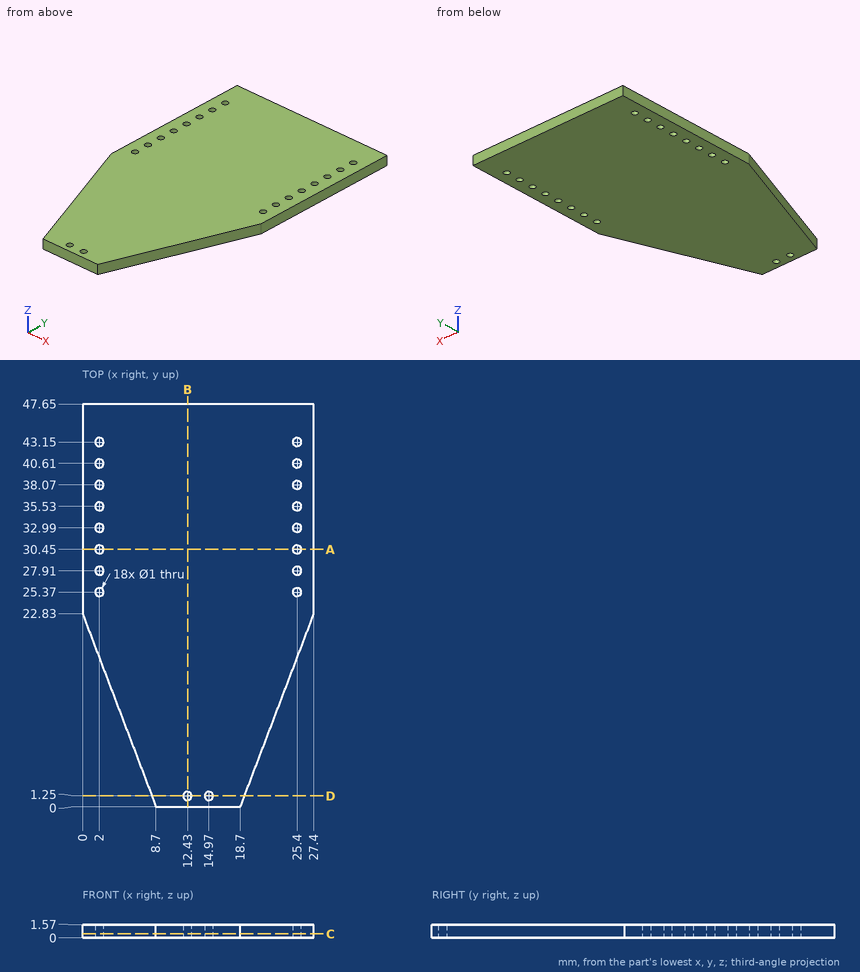
Here's the drawing with two shaded views (mm, measured from the low corner). I have some questions. Coordinates: 2 decimals unless noted, no trailing zeros. Write each loop counter-clockwise with the first axis right and the second up, starting at its lowest first coordinate (ties: lowest second). Pieces come first, ordered by that corner, then holes. Notation, with made-up numbers: (-36, 32.5) - (-5, 32.5) arc R16 ccw to (-5, 53.5) - close; hole circle Ø3 at (40.25, 39.25). An arc over 180 degrees is marked (long way). Return JSON: item names as keys, results as strings.
Q1. If we section it at C-C (z = 0.45): Count the separate pieces of the cut face and the enclosed holes in it, then the cut area to 3 significant figures.
Computed values:
{"separate pieces": "1", "enclosed holes": "18", "area": "1,090 mm2"}
Q2. If we section it at B-B (x = 12.43): Please give me the cut outline in (y, z).
Computed values:
{"outline": "(0, 0) - (0.75, 0) - (0.75, 1.57) - (0, 1.57) - close; (1.75, 0) - (47.65, 0) - (47.65, 1.57) - (1.75, 1.57) - close"}
Q3. If we section it at A-A (y = 30.45): Please give me the cut outline in (x, z), then the cut area to 3 significant figures.
Computed values:
{"outline": "(0, 0) - (1.5, 0) - (1.5, 1.57) - (0, 1.57) - close; (2.5, 0) - (24.9, 0) - (24.9, 1.57) - (2.5, 1.57) - close; (25.9, 0) - (27.4, 0) - (27.4, 1.57) - (25.9, 1.57) - close", "area": "39.9 mm2"}
Q4. Please list where these lines run through material, in increasing order: L1, parallel to X at y = 35.53, z = 1.15; L2, parallel to X at y = 15.5, z = 0.3; L3, parallel to X at y = 10, z = 0.4. Write a range as from..to.
Computed values:
{"L1": "x = 0..1.5, 2.5..24.9, 25.9..27.4", "L2": "x = 2.79..24.61", "L3": "x = 4.89..22.51"}
Q5. If we section it at D-D (y = 1.25): Please give me the cut outline in (x, z).
Computed values:
{"outline": "(8.22, 0) - (11.93, 0) - (11.93, 1.57) - (8.22, 1.57) - close; (12.93, 0) - (14.47, 0) - (14.47, 1.57) - (12.93, 1.57) - close; (15.47, 0) - (19.18, 0) - (19.18, 1.57) - (15.47, 1.57) - close"}
